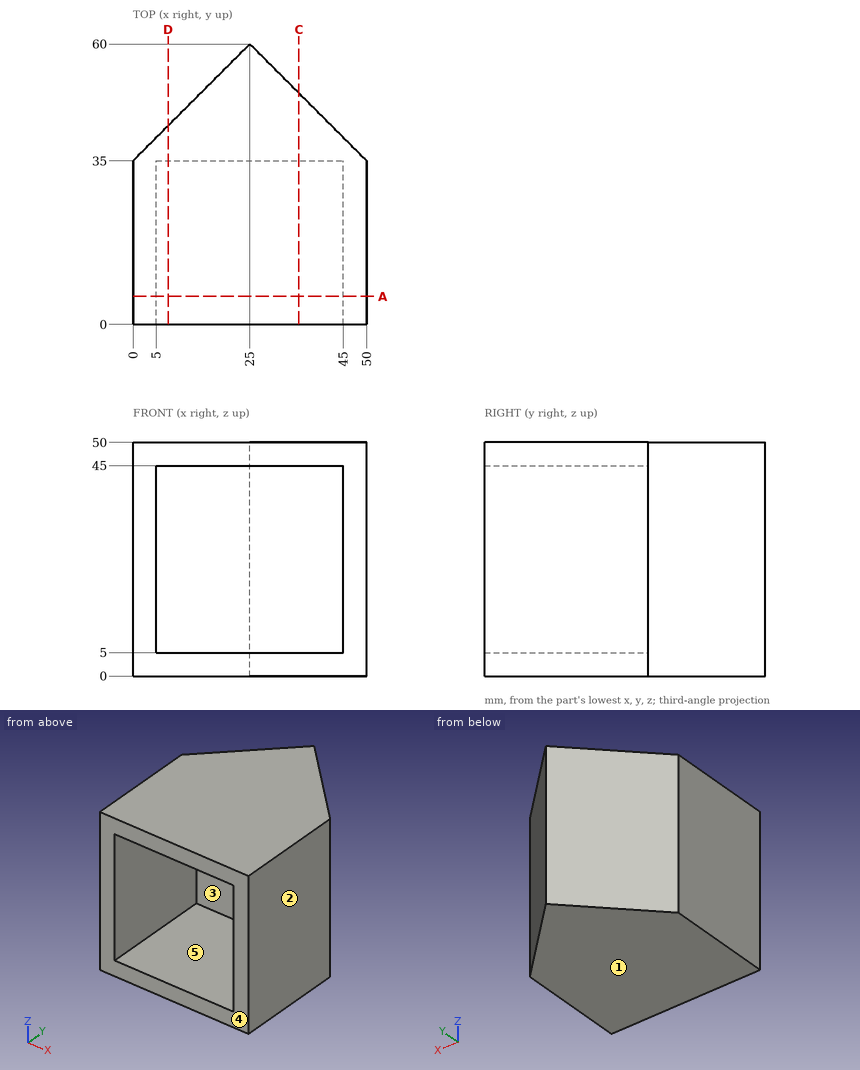
Job drawing, mm, ordinate dimensions from the low corner. One solid piece. A direction names the side the tool comes from. Give positions to 0.01 mm unless a question says otherwise; leave off trailing zeros. Loops run counter-clockwise (first coordinate to the right, second up) from the corner with the lowest first, then second, coordinate; pieces in that order, holes last. Notation, with made-up numbers: (-1, -30) -> (46, -30) arc R15 cw to (46, -24) -> close; hole circle Ø9 at (-29.75, 51). An arc over 180 degrees is marked (long way). Use a Markdown table: item, result. Add a question column.
(1) Slice it at D-D on x = 7.5. List the corners of the cut face in (y, z), and give its area (3 significant figures).
(2) Slice it at A-A on y = 6. List the corners of the cut face in (x, z), and give its area (3 significant figures).
(3) Tool access for the marked faces 4 and 5: list every direction of +Z, -Z, +X, -X, +Y, -Y with a clear straight run to the whole face (end or side of a thin tool).
(4) Wall check: line 1 along Z through (x, y) = (7.5, 33); line 2 along Y through (x, z) = (15, 46). Give the ranges that are in metal, low to high.
(5) Slice it at C-C on x = 35.5. List the corners of the cut face in (y, z), and give its area (4 significant figures).
(6) Drop flat-ended pins along their axis: pin 1 Ø1.5 at (x, z) = (19, 19) entering from -Y; pin 2 Ø2 at (x, z) = (25.5, 21.5) entering from +Y; pin 3 Ø2 at (y, z) = (41, 42.5) entering from -X. Give the stop position or say it passes through.
(7) Mould opens along Z. For the marked faces 1, 2 and 3 say: +Z half, -Z half, draft (parallel to the pull), parting line (faces both ways), or undercut.
Filled sheet:
| question | item | result |
|---|---|---|
| 1 | outline | (0, 0) -> (42.5, 0) -> (42.5, 50) -> (0, 50) -> (0, 45) -> (35, 45) -> (35, 5) -> (0, 5) -> close |
| 1 | area | 725 mm2 |
| 2 | outline | (0, 0) -> (50, 0) -> (50, 50) -> (0, 50) -> close; hole (5, 5) -> (45, 5) -> (45, 45) -> (5, 45) -> close |
| 2 | area | 900 mm2 |
| 3 | face 4 | +Z, -Z, +X, -X, -Y |
| 3 | face 5 | -Y |
| 4 | line 1 | 0 to 5, 45 to 50 |
| 4 | line 2 | 0 to 50 |
| 5 | outline | (0, 0) -> (49.5, 0) -> (49.5, 50) -> (0, 50) -> (0, 45) -> (35, 45) -> (35, 5) -> (0, 5) -> close |
| 5 | area | 1,075 mm2 |
| 6 | pin 1 | y = 35 |
| 6 | pin 2 | y = 60 |
| 6 | pin 3 | x = 5 |
| 7 | face 1 | -Z half |
| 7 | face 2 | draft |
| 7 | face 3 | undercut |
